Read the model definition and answer for the solid it produces. Units are mm, in the model's axes. A direction names the side the tool comes from. Coordinates: 2 decimals unless noted, no trailing zeros. Loops run counter-clockwise (first coordinate to the right, second up) from the corner with the lowest first, then second, coordinate; pieces in that order, holes last.
from build123d import *

# Parameters (mm, degrees)
BOSS_EXTRU_1_DEPTH = 5


with BuildPart() as part:
    # Esquisse1 → Boss.-Extru.1 (new body)
    with BuildSketch(Plane.XY):
        with BuildLine():
            Line((55, 95), (55, 35))
            ThreePointArc((55, 35), (53.535533906, 31.464466094), (50, 30))
            Line((50, 30), (25, 30))
            ThreePointArc((25, 30), (20, 25), (25, 20))
            Line((25, 20), (50, 20))
            ThreePointArc((50, 20), (53.535533906, 18.535533906), (55, 15))
            Line((55, 15), (55, 5))
            ThreePointArc((55, 5), (53.535533906, 1.464466094), (50, 0))
            Line((50, 0), (5, 0))
            ThreePointArc((5, 0), (1.464466094, 1.464466094), (0, 5))
            Line((0, 5), (0, 95))
            ThreePointArc((0, 95), (1.464466094, 98.535533906), (5, 100))
            Line((5, 100), (50, 100))
            ThreePointArc((50, 100), (53.535533906, 98.535533906), (55, 95))
        make_face()
    extrude(amount=BOSS_EXTRU_1_DEPTH)


solid = part.part
Item 1: A cutting plane is placed at A-A on x = 38.5. Determine the outline of the cut face in (y, z).
Numbers:
outline: (0, 0) - (20, 0) - (20, 5) - (0, 5) - close; (30, 0) - (100, 0) - (100, 5) - (30, 5) - close
Item 2: Which of the six approach directions +Z, -Z, +X, -X, +Y, -Y give full straight-line access (tool end or side, diameter ignored) to faces 5 (the face through (0, 49, 2)), 6 (the face through (54, 32, 2))?
Numbers:
face 5: +Z, -Z, -X, +Y, -Y
face 6: +Z, -Z, +X
Item 3: Find the intervals of material crossed by line 1 along Y through (x, z) = (31, 3.2); line 2 along Y through (x, z) = (24, 3.3); line 3 along X through (y, z) = (28, 0.25), in increasing order.
Numbers:
line 1: y = 0 to 20, 30 to 100
line 2: y = 0 to 20.1, 29.9 to 100
line 3: x = 0 to 21
Item 4: Determine the mould class of faces 1 (the face through (28, 51, 5)), 2 (the face through (38, 30, 2)), 3 (the face through (20, 25, 2)), 4 (the face through (2, 1, 2)) for opening direction Y: released by +Y, released by -Y, zero draft, split by the parting line, or undercut.
Numbers:
face 1: zero draft
face 2: undercut
face 3: undercut
face 4: released by -Y
Item 5: Given pin 1 (3 mm diameter, centred on x = 25, y = 35.5, fed in from -Z), flat-ended and moving along its own axis, determine where the tip first touches the part or whether it passes through.
Numbers:
pin 1: stops at z = 0
Item 6: A cutting plane is placed at C-C on y = 25. Determine the outline of the cut face in (x, z).
Numbers:
outline: (0, 0) - (20, 0) - (20, 5) - (0, 5) - close
Item 7: A cutting plane is placed at B-B on z = 0.9. Determine the outline of the cut face in (x, y).
Numbers:
outline: (0, 5) arc R5 ccw to (5, 0) - (50, 0) arc R5 ccw to (55, 5) - (55, 15) arc R5 ccw to (50, 20) - (25, 20) arc R5 cw to (25, 30) - (50, 30) arc R5 ccw to (55, 35) - (55, 95) arc R5 ccw to (50, 100) - (5, 100) arc R5 ccw to (0, 95) - close
